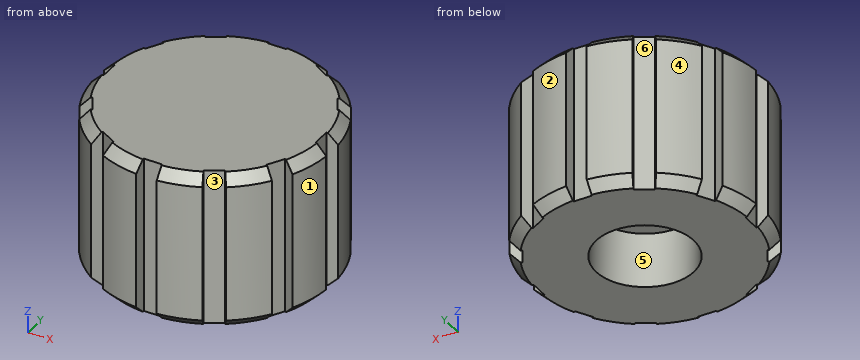
```python
from build123d import *

# Parameters (mm, degrees)
SKETCH002_R        = 12
PAD002_DEPTH       = 16
CHAMFER_SIZE       = 1
POCKET_DEPTH       = 75.047652
POCKET_DEPTH_BACK  = 91.047652
POLARPATTERN_COUNT = 12
SKETCH_R           = 5
POCKET001_DEPTH    = 5.6
POCKET002_DEPTH    = 14


with BuildPart() as part:
    # Sketch002 → Pad002 (new body)
    with BuildSketch(Plane.XY):
        Circle(SKETCH002_R)
    extrude(amount=PAD002_DEPTH)

    # Chamfer
    chamfer_edges = [part.edges().sort_by_distance(p)[0] for p in [
        (-12, 0, 16),
        (-12, 0, 0),
    ]]
    chamfer(chamfer_edges, length=CHAMFER_SIZE)

    # Sketch003 → Pocket (cut, two sides)
    with BuildSketch(Plane.XY) as pocket_sk:
        Polygon((-1.058613, 12.1), (-0.944878, 10.8), (0.944878, 10.8), (1.058613, 12.1), align=None)
    pocket = extrude(amount=-POCKET_DEPTH, mode=Mode.SUBTRACT) + extrude(pocket_sk.sketch, amount=POCKET_DEPTH_BACK, mode=Mode.SUBTRACT)

    # PolarPattern: Pocket ×12 about axis
    polarpattern_axis = Axis((0, 0, 0), (0, 0, 1))
    for i in range(1, POLARPATTERN_COUNT):
        add(pocket.rotate(polarpattern_axis, i * 360 / POLARPATTERN_COUNT), mode=Mode.SUBTRACT)

    # Sketch → Pocket001 (cut)
    with BuildSketch(Plane.XY):
        Circle(SKETCH_R)
    extrude(amount=POCKET001_DEPTH, mode=Mode.SUBTRACT)

    # Sketch004 → Pocket002 (cut)
    with BuildSketch(Plane.XY):
        with BuildLine():
            ThreePointArc((-1.55, -2.626785), (3.05, 0), (-1.55, 2.626785))
            Line((-1.55, 2.626785), (-1.55, -2.626785))
        make_face()
    extrude(amount=POCKET002_DEPTH, mode=Mode.SUBTRACT)


solid = part.part
```
Design review of the part built by this model. Coordinates are the model's own, in mm. Face numbers are marked on the shaded views. A direction names the side the tool comes from. Coordinates: 2 decimals unless noted, no trailing zeros. Loops run counter-clockwise (first coordinate to the right, second up) from the corner with the lowest first, then second, coordinate; pieces in that order, holes last.
Q1. The part is to be moulded in two halves that separate along Y. For the marked faces 1, 2 and 3, say which applies: +Y half, -Y half, draft (parallel to the pull), parting line (faces both ways), or undercut.
Reported:
face 1: -Y half
face 2: +Y half
face 3: undercut
Q2. We need section A-A on y = 0. State the section outline as (x, z) points, and give its area (3 significant figures).
Reported:
outline: (-10.8, 0) - (-5, 0) - (-5, 5.6) - (-1.55, 5.6) - (-1.55, 14) - (3.05, 14) - (3.05, 5.6) - (5, 5.6) - (5, 0) - (10.8, 0) - (10.8, 16) - (-10.8, 16) - close
area: 251 mm2
Q3. Tool access review of the marked faces 4, 5 and 6: name each direction out of +Z, -Z, +X, -X, +Y, -Y from which nothing blocks a thin tool from reaching the whole face with its end or side.
Reported:
face 4: +Z, -Z, -X, +Y
face 5: -Z
face 6: +Z, -Z
Q4. We need section B-B on x = 0. State the section outline as (y, z) points.
Reported:
outline: (-10.8, 0) - (-5, 0) - (-5, 5.6) - (-3.05, 5.6) - (-3.05, 14) - (3.05, 14) - (3.05, 5.6) - (5, 5.6) - (5, 0) - (10.8, 0) - (10.8, 16) - (-10.8, 16) - close
Q5. For pin 1 (0.6 mm diameter, centred on x = 0, z = 10.5, fed in from +Y); pin 2 (6 mm diameter, centred on y = -5.5, z = 11.5, fed in from -X); pin 3 (3.5 mm diameter, centred on x = 0, y = 0, fed in from -Z), all flat-tipped, find the tip position at first contact; note any pin that passes through.
Reported:
pin 1: stops at y = 10.8
pin 2: stops at x = -11.74
pin 3: stops at z = 5.6
Q6. To check wall thickness, follow line 1 (Y direction, x = 0, z = 12); line 2 (X direction, y = -5, z = 13); line 3 (Y direction, x = 9, z = 0.75). State the ranges of each line that lie inside material, in increasing order.
Reported:
line 1: y = -10.8 to -3.05, 3.05 to 10.8
line 2: x = -10.91 to -10.72, -9.58 to 9.58, 10.72 to 10.91
line 3: y = -7.55 to -6.3, -6.01 to 6.01, 6.3 to 7.55
